Verification items for the finished model (mm, model axes). Face numbers are marked on the shaded views. A direction names the side the tool comes from. Round coordinates to 2 decimals unless told otherwise and drop trailing zeros. Write each loop counter-clockwise with the first axis right and the second up, starting at its lowest first coordinate (ties: lowest second). Pieces come first, ordered by that corner, then holes.
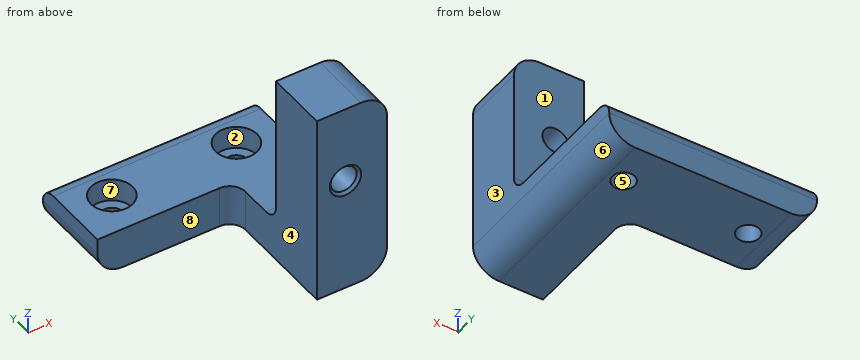
from build123d import *

# Parameters (mm, degrees)
SKETCH1_W                                           = 40
SKETCH1_H                                           = 37.5
BOSS_EXTRUDE1_DEPTH                                 = 40
CUT_EXTRUDE1_REACH                                  = 61.595
SKETCH2_W                                           = 29.5
SKETCH2_H                                           = 28
FILLET1_R                                           = 3
M6_TAPPED_HOLE1_D                                   = 5
M6_TAPPED_HOLE1_CSINK_D                             = 6.05
M6_TAPPED_HOLE1_CSINK_ANGLE                         = 90
FILLET2_R                                           = 5
CUT_EXTRUDE2_REACH                                  = 50.493
SKETCH7_W                                           = 13
SKETCH7_H                                           = 29.5
CUT_EXTRUDE3_REACH                                  = 50.493
SKETCH8_W                                           = 29.5
SKETCH8_H                                           = 37
CUT_EXTRUDE4_REACH                                  = 61.595
SKETCH9_W                                           = 8
SKETCH9_H                                           = 23.997787144
FILLET5_R                                           = 3
CBORE_FOR_M4_HEX_SOCKET_HEAD_CAP_SCREW1_D           = 4.3
CBORE_FOR_M4_HEX_SOCKET_HEAD_CAP_SCREW1_CBORE_D     = 8
CBORE_FOR_M4_HEX_SOCKET_HEAD_CAP_SCREW1_CBORE_DEPTH = 4.4


with BuildPart() as part:
    # Sketch1 → Boss-Extrude1 (new body)
    with BuildSketch(Plane(origin=(0, 0, 0), x_dir=(1, 0, 0), z_dir=(0, 1, 0))):
        Rectangle(SKETCH1_W, SKETCH1_H)
    extrude(amount=-BOSS_EXTRUDE1_DEPTH)

    # Sketch2 → Cut-Extrude1 (cut, up to next)
    with BuildSketch(Plane(origin=(20, 0, 0), x_dir=(0, 0, -1), z_dir=(1, 0, 0)), mode=Mode.PRIVATE) as cut_extrude1_sk1:
        with Locations((-4, -14)):
            Rectangle(SKETCH2_W, SKETCH2_H)
    cut_extrude1_tool1 = extrude(cut_extrude1_sk1.sketch, amount=-CUT_EXTRUDE1_REACH, mode=Mode.PRIVATE) & part.part
    add(cut_extrude1_tool1.solids().sort_by_distance((20, -14, 4))[0], mode=Mode.SUBTRACT)

    # Fillet1
    fillet1_edges = [part.edges().sort_by_distance(p)[0] for p in [
        (0, 0, -10.75),
        (0, -28, -10.75),
    ]]
    fillet(fillet1_edges, radius=FILLET1_R)

    # M6 Tapped Hole1 (through all)
    with Locations(Plane(origin=(0, -40, 0), x_dir=(-1, 0, 0), z_dir=(0, -1, 0))):
        with Locations((-12, -3.75)):
            CounterSinkHole(M6_TAPPED_HOLE1_D / 2, M6_TAPPED_HOLE1_CSINK_D / 2, counter_sink_angle=M6_TAPPED_HOLE1_CSINK_ANGLE)

    # Fillet2
    fillet2_edges = [part.edges().sort_by_distance(p)[0] for p in [
        (20, -20, -18.75),
        (20, -34, 18.75),
        (-20, -34, 18.75),
        (-20, -20, -18.75),
    ]]
    fillet(fillet2_edges, radius=FILLET2_R)

    # Sketch7 → Cut-Extrude2 (cut, up to next)
    with BuildSketch(Plane(origin=(0, 0, 0), x_dir=(1, 0, 0), z_dir=(0, 1, 0)), mode=Mode.PRIVATE) as cut_extrude2_sk1:
        with Locations((0, -4)):
            Rectangle(SKETCH7_W, SKETCH7_H)
    cut_extrude2_tool1 = extrude(cut_extrude2_sk1.sketch, amount=-CUT_EXTRUDE2_REACH, mode=Mode.PRIVATE) & part.part
    add(cut_extrude2_tool1.solids().sort_by_distance((0, 0, 4))[0], mode=Mode.SUBTRACT)

    # Sketch8 → Cut-Extrude3 (cut, up to next)
    with BuildSketch(Plane(origin=(0, 0, 0), x_dir=(0, 0, -1), z_dir=(1, 0, 0)), mode=Mode.PRIVATE) as cut_extrude3_sk1:
        with Locations((-4, -21.5)):
            Rectangle(SKETCH8_W, SKETCH8_H)
    cut_extrude3_tool1 = extrude(cut_extrude3_sk1.sketch, amount=-CUT_EXTRUDE3_REACH, mode=Mode.PRIVATE) & part.part
    add(cut_extrude3_tool1.solids().sort_by_distance((0, -21.5, 4))[0], mode=Mode.SUBTRACT)

    # Cut-Extrude4: up to this face of the body (flat: up to its plane)
    cut_extrude4_end = Plane(part.part.faces().sort_by_distance((6.5, -33.963805531, 3.923597235))[0])
    # Sketch9 → Cut-Extrude4 (cut, up to the picked face)
    with BuildSketch(Plane.ZY.offset(20), mode=Mode.PRIVATE) as cut_extrude4_sk1:
        with Locations((-14.75, -28.001106428)):
            Rectangle(SKETCH9_W, SKETCH9_H)
    cut_extrude4_tool1 = split(extrude(cut_extrude4_sk1.sketch, amount=-CUT_EXTRUDE4_REACH, mode=Mode.PRIVATE), bisect_by=cut_extrude4_end, keep=Keep.BOTH, mode=Mode.PRIVATE)
    add(cut_extrude4_tool1.solids().sort_by(Axis((-20, -28.001106, -14.75), (1, 0, 0)))[0], mode=Mode.SUBTRACT)

    # Fillet5
    fillet5_edges = [part.edges().sort_by_distance(p)[0] for p in [
        (6.5, -16.002212856, -14.75),
    ]]
    fillet(fillet5_edges, radius=FILLET5_R)

    # CBORE for M4 Hex Socket Head Cap Screw1 (through all)
    with Locations(Plane.XY.offset(-10.75)):
        with Locations((-12, -8.001106428), (12, -8.001106428)):
            CounterBoreHole(CBORE_FOR_M4_HEX_SOCKET_HEAD_CAP_SCREW1_D / 2, CBORE_FOR_M4_HEX_SOCKET_HEAD_CAP_SCREW1_CBORE_D / 2, CBORE_FOR_M4_HEX_SOCKET_HEAD_CAP_SCREW1_CBORE_DEPTH)


solid = part.part
Q1. Sectioned sample at D-D (y = -11). Enter the section's corners in (x, z), plus the area to 3 significant figures.
Recorded:
outline: (-20, -13.75) arc R5 ccw to (-15, -18.75) - (15, -18.75) arc R5 ccw to (20, -13.75) - (20, -10.75) - (14.65, -10.75) - (14.65, -15.15) - (9.35, -15.15) - (9.35, -10.75) - (-9.35, -10.75) - (-9.35, -15.15) - (-14.65, -15.15) - (-14.65, -10.75) - (-20, -10.75) - close
area: 263 mm2
Q2. Tool access check on the marked faces 1, 2, 3 and 4. Record the directions out of +Z, -Z, +X, -X, +Y, -Y that give a thin tool (end or side, any length) a straight path to the whole face; none if there is none.
Recorded:
face 1: +Z, +X, -X, +Y
face 2: +Z
face 3: +Z, -Z, +X, +Y, -Y
face 4: +Z, -Z, -X, -Y
Q3. Depth check by flat-ended pin: P1, Ø8, axis at x = 13, z = 14, coming from the +Y side; P2, Ø4, axis at x = 11, y = -7.5, coming from the +Z side; P3, Ø3, axis at x = -11, z = -12, coming from the +Y side. Enter the tip coordinate at first touch or a pass-through.
Recorded:
P1: stops at y = -28
P2: stops at z = -15.15
P3: stops at y = -0.01
Q4. Release check for a two-part mould opening along Y. For the marked faces 5, 6, 7 and 8 record: released by +Y, released by -Y, zero draft, split by the parting line, or undercut.
Recorded:
face 5: undercut
face 6: zero draft
face 7: undercut
face 8: released by -Y
Q5. Sectioned sample at B-B (y = -33). Enter the section's corners in (x, z), plus the area to 3 significant figures.
Recorded:
outline: (6.5, -18.75) - (15, -18.75) arc R5 ccw to (20, -13.75) - (20, 13.75) arc R5 ccw to (15, 18.75) - (6.5, 18.75) - close; hole circle Ø5 at (12, 3.75)
area: 476 mm2
Q6. Sectioned sample at C-C (x = 12). Enter the section's corners in (y, z) (3 decimals), plus the area to 3 significant figures.
Recorded:
outline: (-40, -18.75) - (-10.151, -18.75) - (-10.151, -15.15) - (-12.001, -15.15) - (-12.001, -10.75) - (-25, -10.75) arc R3 cw to (-28, -7.75) - (-28, 1.25) - (-39.475, 1.25) - (-40, 0.725) - close; (-40, 6.775) - (-39.475, 6.25) - (-28, 6.25) - (-28, 18.75) - (-40, 18.75) - close; (-5.851, -18.75) - (0, -18.75) - (0, -13.75) arc R3 ccw to (-3, -10.75) - (-4.001, -10.75) - (-4.001, -15.15) - (-5.851, -15.15) - close
area: 563 mm2
Q7. Sectioned sample at A-A (z = 3.75). Enter the section's corners in (x, y) (3 decimals), plus the area to 3 significant figures.
Recorded:
outline: (6.5, -40) - (8.975, -40) - (9.5, -39.475) - (9.5, -28) - (6.5, -28) - close; (14.5, -39.475) - (15.025, -40) - (20, -40) - (20, -28) - (14.5, -28) - close
area: 102 mm2
Q8. Material ranges on line 1 along Y through (x, z) = (-12, -17); line 2 along Z through (x, y) = (12, -35); line 3 along Y through (x, z) = (12, -16), recorded low to high.
Recorded:
line 1: y = -16 to -10.15, -5.85 to 0
line 2: z = -18.75 to 1.25, 6.25 to 18.75
line 3: y = -40 to -10.15, -5.85 to 0
